Geometry: see drawing. Coordinates: mm, zero at the bounding-box minimum. Give positions to 0.01 mm unless a question says otherwise; leave off trailing zeros. Loops run counter-clockwise (first coordinate to the right, second up) from the corner with the lowest first, then second, coordinate; pieces in that order, holes last. Notation, with made-up numbers: (5.25, 86.5) - (44.25, 86.5) arc R22 cw to (44.25, 94.5) - close; hole circle Ø9 at (0.25, 28). An arc over 180 degrees is marked (long way). Use one line per item in the form item = value.
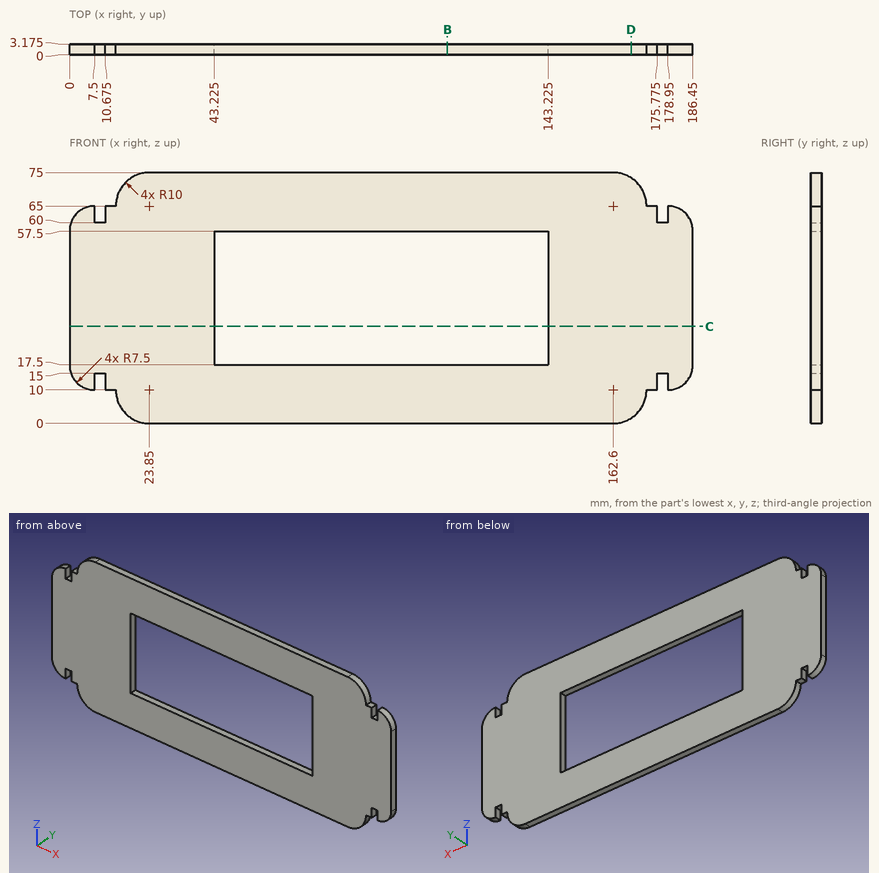
(1) Cut plane D-D (x = 168). Return the cut outline in (y, z) (3 decimals).
Solution:
outline = (0, 1.583) - (3.175, 1.583) - (3.175, 73.417) - (0, 73.417) - close
(2) Cut plane B-B (x = 113). Return the cut outline in (y, z) (3 decimals), plus the area to 3 significant figures.
Solution:
outline = (0, 0) - (3.175, 0) - (3.175, 17.5) - (0, 17.5) - close; (0, 57.5) - (3.175, 57.5) - (3.175, 75) - (0, 75) - close
area = 111 mm2
(3) Pin query (flat end, axial travel): P1, Ø1, axis at x = 174.5, y = 1, coming from the +Z side; P2, Ø1, axis at y = 1.5, z = 12.5, coming from the -X side; P3, Ø1.6, axis at x = 12.5, y = 2, coming from the -Z side. Return the tip coordinate at first contact, or that it passes through.
Solution:
P1 = 65
P2 = 1.5
P3 = 10
(4) Cut plane C-C (z = 29). Return the cut outline in (x, y) (3 decimals), plus the area to 3 significant figures.
Solution:
outline = (0, 0) - (43.225, 0) - (43.225, 3.175) - (0, 3.175) - close; (143.225, 0) - (186.45, 0) - (186.45, 3.175) - (143.225, 3.175) - close
area = 274 mm2
(5) Material intervals for L1, parallel to Z at x = 103, y = 2.95; L2, parallel to X at y = 1.5, z = 51.5 (3 decimals); L3, parallel to X at y = 0.9, z = 14 (3 decimals), sorted ascending. Write a range as from..to.
Solution:
L1 = 0..17.5, 57.5..75
L2 = 0..43.225, 143.225..186.45
L3 = 0.867..7.5, 10.675..175.775, 178.95..185.583
